Design review of the part built by this model. Coordinates are the model's own, in mm. Face numbers are marked on the shaded views. Coordinates: 2 decimals unless noted, no trailing zeros. Order: outer loops, then holes, each group sorted by start corner. A loop starts at its lowest first (then second) coordinate and runs counter-clockwise, first axis right, second up. Notation, with made-up numbers: M -37.75,-11 L -15.75,-11 A22 ccw -15.75,9 Z; hole C -15.5,43 d8. An arc over 180 degrees is marked long. Answer as a JSON object with one key per item and string values.
from build123d import *

# Parameters (mm, degrees)
BOSS_EXTRUDE1_DEPTH = 254
CUT_EXTRUDE1_DEPTH  = 2878.185
SKETCH6_R           = 217.8177
CUT_EXTRUDE2_DEPTH  = 2878.1850001
SKETCH7_W           = 88.9
SKETCH7_H           = 50.8
BOSS_EXTRUDE2_DEPTH = 38.1
BOSS_EXTRUDE3_DEPTH = 9.525
BOSS_EXTRUDE4_DEPTH = 12.7


with BuildPart() as part:
    # Sketch3 → Boss-Extrude1 (new body)
    with BuildSketch(Plane(origin=(0, 0, 0), x_dir=(0, 0, -1), z_dir=(1, 0, 0))):
        with BuildLine():
            Line((2844.8, 44.45), (2607.629412658, 0))
            Line((2607.629412658, 0), (0, 0))
            Line((0, 0), (0, 53.975))
            Line((0, 53.975), (2844.8, 53.975))
            Line((2844.8, 53.975), (2844.8, 50.165))
            ThreePointArc((2844.8, 50.165), (2867.250640303, 59.464359697), (2876.55, 81.915))
            Line((2876.55, 81.915), (2877.185, 81.915))
            ThreePointArc((2877.185, 81.915), (2867.699653109, 59.015346891), (2844.8, 49.53))
            Line((2844.8, 49.53), (2844.8, 44.45))
        make_face()
    extrude(amount=-BOSS_EXTRUDE1_DEPTH)

    # Sketch5 → Cut-Extrude1 (cut, through all)
    with BuildSketch(Plane.XY):
        with BuildLine():
            Line((0, 65.7225), (0, 81.915))
            Line((0, 81.915), (-16.1925, 81.915))
            ThreePointArc((-16.1925, 81.915), (-4.742673446, 77.172326554), (0, 65.7225))
        make_face()
        with BuildLine():
            Line((-254, 65.7225), (-254, 81.915))
            Line((-254, 81.915), (-237.8075, 81.915))
            ThreePointArc((-237.8075, 81.915), (-249.257326554, 77.172326554), (-254, 65.7225))
        make_face()
    extrude(amount=-CUT_EXTRUDE1_DEPTH, mode=Mode.SUBTRACT)

    # Sketch6 → Cut-Extrude2 (cut, through all)
    with BuildSketch(Plane.XY):
        with Locations((-127, -191.7827)):
            Circle(SKETCH6_R)
    extrude(amount=-CUT_EXTRUDE2_DEPTH, mode=Mode.SUBTRACT)

    # Sketch7 → Boss-Extrude2 (add)
    with BuildSketch(Plane(origin=(0, 53.975, 0), x_dir=(1, 0, 0), z_dir=(0, 1, 0))):
        with Locations((-127, 25.4)):
            Rectangle(SKETCH7_W, SKETCH7_H)
    extrude(amount=BOSS_EXTRUDE2_DEPTH)

    # Sketch8 → Boss-Extrude3 (add)
    with BuildSketch(Plane(origin=(0, 53.975, 0), x_dir=(1, 0, 0), z_dir=(0, 1, 0))):
        Polygon((-34.219914215, 88.9), (-34.219914215, 82.55), (-25.075914215, 82.55), (-25.075914215, 63.5), (-34.219914215, 63.5), (-34.219914215, 50.8), (-72.319914215, 50.8), (-72.319914215, 63.5), (-148.900914215, 63.5), (-148.900914215, 82.55), (-40.569914215, 82.55), (-40.569914215, 88.9), align=None)
    extrude(amount=BOSS_EXTRUDE3_DEPTH)

    # Sketch9 → Boss-Extrude4 (add)
    with BuildSketch(Plane(origin=(0, 63.5, 0), x_dir=(1, 0, 0), z_dir=(0, 1, 0))):
        Polygon((-72.319914215, 50.8), (-40.569914215, 82.55), (-40.569914215, 88.9), (-34.219914215, 88.9), (-34.219914215, 50.8), align=None)
    extrude(amount=BOSS_EXTRUDE4_DEPTH)


solid = part.part
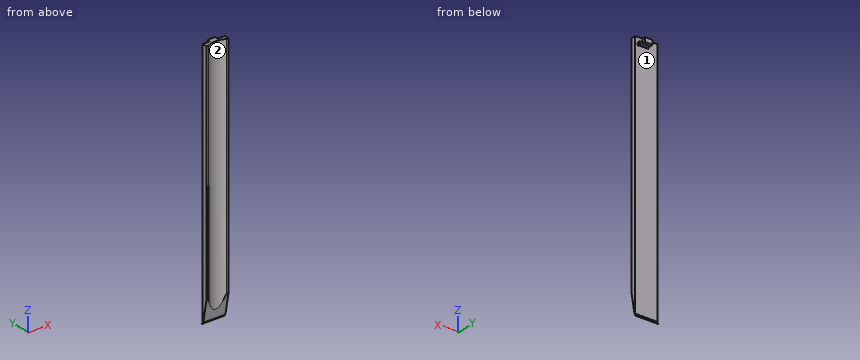
1) Insertion check: pin 1 Ø7 at (x, y) = (-38, 64.5) entering from -Z; pin 2 Ø1.5 at (y, z) = (50, -1756) entering from +X; pin 3 Ø2.5 at (x, y) = (-30.5, 56.5) entering from -Z; pin 4 Ø7 at (y, z) = (61, -85.5) entering from -X. Each pin has a flat end and moves straight along its axis. Give the tip position at first contact, or say it passes through.
Taken from the geometry:
{"pin 1": "stops at z = -2874.04", "pin 2": "stops at x = 0", "pin 3": "stops at z = -2866.36", "pin 4": "stops at x = -148.9"}
2) Mouldability with a two-part tool opening along X and no side actions: class the marked faces 1 and 2 as released by +X, released by -X, zero draft, split by the parting line, or undercut.
Taken from the geometry:
{"face 1": "zero draft", "face 2": "undercut"}
3) Add section A-A (z = -871). State the section outline as (x, y) points (3 decimals), and give its area (3 significant figures).
Taken from the geometry:
{"outline": "M -254,0 L -230.266,0 A217.818 cw -23.734,0 L 0,0 L 0,53.975 L -254,53.975 Z", "area": "10,100 mm2"}
4) To check wall thickness, follow L1, parallel to Y at x = -129.5, z = -1976 (3 decimals); L2, parallel to Z at x = -82.5, y = 66; L3, parallel to Z at x = -35, y = 74. State the ranges of each line that lie inside material, in increasing order.
Taken from the geometry:
{"L1": "y = 26.021 to 53.975", "L2": "z = -2873 to -2872.27", "L3": "z = -2876.2 to -2875.55, -88.9 to -50.8"}
5) Add section B-B (z = -2664). State the section outline as (x, y) points (3 decimals).
Taken from the geometry:
{"outline": "M -254,10.565 L -207.623,10.565 A217.818 cw -46.377,10.565 L 0,10.565 L 0,53.975 L -254,53.975 Z"}
